Geometry: final body of the model. Coordinates: model frame, mm. A direction names the side the tool comes from. Give positions to 0.01 mm unless a question says otherwise; leave off trailing zeros. Loops run counter-clockwise (first coordinate to the right, second up) from the corner with the lowest first, then second, coordinate; pieces in that order, holes last. Notation, with made-up numbers: (3.25, -24.75) - (40.25, -24.75) arc R13 ccw to (40.25, -19.75) - close; hole circle Ø9 at (41.25, 47.5). An arc over 180 degrees is marked (long way). Answer in a Markdown table with one row per item.
from build123d import *

# Parameters (mm, degrees)
SFAZOWANIE1_SIZE           = 0.35
ZAOKR_GLENIE1_R            = 0.35
WYTNIJ_WYCI_GNI_CIE1_DEPTH = 3


with BuildPart() as part:
    # Szkic1 → Obrót1 (revolve)
    with BuildSketch(Plane.XY):
        Polygon((0, 0), (0, 3.5), (-4, 3.5), (-4, 2), (-14, 2), (-14, 0), align=None)
    revolve(axis=Axis((-123.158940217, 0, 0), (1, 0, 0)))

    # Sfazowanie1
    sfazowanie1_edges = [part.edges().sort_by_distance(p)[0] for p in [
        (-14, -2, 0),
    ]]
    chamfer(sfazowanie1_edges, length=SFAZOWANIE1_SIZE)

    # Zaokrąglenie1
    zaokr_glenie1_edges = [part.edges().sort_by_distance(p)[0] for p in [
        (0, -3.5, 0),
    ]]
    fillet(zaokr_glenie1_edges, radius=ZAOKR_GLENIE1_R)

    # Szkic2 → Wytnij-wyciągnięcie1 (cut)
    with BuildSketch(Plane(origin=(0, 0, 0), x_dir=(0, 0, -1), z_dir=(1, 0, 0))):
        Polygon((1.732050808, 0), (0.866025404, 1.5), (-0.866025404, 1.5), (-1.732050808, 0), (-0.866025404, -1.5), (0.866025404, -1.5), align=None)
    extrude(amount=-WYTNIJ_WYCI_GNI_CIE1_DEPTH, mode=Mode.SUBTRACT)


solid = part.part
Q1. Reachability of faces 4 (the flat face through (-1, 1.5, 0)), 5 (the flat face through (-14, 0, 0)), 6 (the flat face through (-4, 2, -2)) from +Z, -Z, +X, -X, +Y, -Y: full face, straight path, thin tool, end or side. Return the list, or none.
Check values:
| item | result |
|---|---|
| face 4 | +X |
| face 5 | +Z, -Z, -X, +Y, -Y |
| face 6 | -X |
Q2. Draft query along Z for faces 1 (the cylindrical face through (-2.201, 3.233, -1.341)), 2 (the flat face through (-1.479, -0.76, -1.293)), 3 (the flat face through (0, -1.4, -1.4)). Return one class per face: pulls with the +Z half, pulls with the -Z half, needs draft (parallel to the pull), parting line crosses it, or undercut.
Check values:
| item | result |
|---|---|
| face 1 | parting line crosses it |
| face 2 | undercut |
| face 3 | needs draft |
Q3. First-contact query: pin 1 (1.5 mm diameter, centred on x = -8.5, y = -0.5, fed in from -Z); pin 2 (1.5 mm diameter, centred on x = -8, z = -3, fed in from +Y); pin 3 (2 mm diameter, centred on x = -8, z = 1.5, fed in from -Y); pin 4 (4 mm diameter, centred on x = -10, y = 2, fed in from +Z). Flat tips, straight axial feed; report the tip coordinate or a pass-through.
Check values:
| item | result |
|---|---|
| pin 1 | z = -2 |
| pin 2 | through |
| pin 3 | y = -1.94 |
| pin 4 | z = 2 |
Q4. Material intervals for line 1 along X through (y, z) = (-1.75, -2.25); line 2 along Z through (x, y) = (-4.5, -1); line 3 along Z through (x, y) = (-1.5, 0.75), sorted ascending.
Check values:
| item | result |
|---|---|
| line 1 | -4 to 0 |
| line 2 | -1.73 to 1.73 |
| line 3 | -3.42 to -1.3, 1.3 to 3.42 |
Q5. Cut plane A-A (x = -0.75). Output: boundary loops of the cut face in (y, z).
Check values:
| item | result |
|---|---|
| outline | circle Ø7 at (0, 0); hole (-1.5, -0.87) - (0, -1.73) - (1.5, -0.87) - (1.5, 0.87) - (0, 1.73) - (-1.5, 0.87) - close |
Q6. Cut plane C-C (x = -6.5). Output: boundary loops of the cut face in (y, z), and give its area (3 significant figures).
Check values:
| item | result |
|---|---|
| outline | circle Ø4 at (0, 0) |
| area | 12.6 mm² |
Q7. Cut plane B-B (z = 0). Output: boundary loops of the cut face in (x, y).
Check values:
| item | result |
|---|---|
| outline | (-14, -1.65) - (-13.65, -2) - (-4, -2) - (-4, -3.5) - (-0.35, -3.5) arc R0.35 ccw to (0, -3.15) - (0, -1.5) - (-3, -1.5) - (-3, 1.5) - (0, 1.5) - (0, 3.15) arc R0.35 ccw to (-0.35, 3.5) - (-4, 3.5) - (-4, 2) - (-13.65, 2) - (-14, 1.65) - close |
